Read the model definition and answer for the solid it produces. Units are mm, in the model's axes. A direction names the side the tool comes from. Coordinates: 2 decimals unless noted, no trailing zeros. Order: outer loops, then holes, each group sorted by start corner. A loop starts at its lowest first (then second) coordinate and runs counter-clockwise, first axis right, second up. Notation, with made-up numbers: (-22, 75) - (10, 75) arc R22 cw to (10, 110) - close; hole circle Ø10 at (42.25, -12.5). An arc over 180 degrees is marked (long way). Answer as a JSON object with one key per item and string values. Group by question number.
from build123d import *

# Parameters (mm, degrees)
ESQUISSE1_W        = 95
ESQUISSE1_H        = 75
BOSS_EXTRU_1_DEPTH = 5
BOSS_EXTRU_2_DEPTH = 25
ESQUISSE3_W        = 4.5
ESQUISSE3_H        = 7.5
BOSS_EXTRU_3_DEPTH = 90


with BuildPart() as part:
    # Esquisse1 → Boss.-Extru.1 (new body)
    with BuildSketch(Plane.XY):
        with Locations((47.5, 37.5)):
            Rectangle(ESQUISSE1_W, ESQUISSE1_H)
    extrude(amount=BOSS_EXTRU_1_DEPTH)

    # Esquisse2 → Boss.-Extru.2 (add)
    with BuildSketch(Plane.XY.offset(5)):
        Polygon((0, 70), (0, 75), (95, 75), (95, 0), (0, 0), (0, 5), (90, 5), (90, 70), align=None)
    extrude(amount=BOSS_EXTRU_2_DEPTH)

    # Esquisse3 → Boss.-Extru.3 (add)
    with BuildSketch(Plane.ZY.offset(-90)):
        with Locations((27.75, 66.25)):
            Rectangle(ESQUISSE3_W, ESQUISSE3_H)
        with Locations((27.75, 8.75)):
            Rectangle(ESQUISSE3_W, ESQUISSE3_H)
    extrude(amount=BOSS_EXTRU_3_DEPTH)


solid = part.part
1. For faces 1 (the flat face through (47, 38, 0)), 2 (the flat face through (46, 9, 25.5)), 3 (the flat face through (46, 62.5, 28)), determine the directions among +Z, -Z, +X, -X, +Y, -Y from which every point of the face is accessible in a straight line to the end or side of a thin tool.
2. Straight lines are drawn through the part: L1, parallel to Y at x = 61, z = 17.5; L2, parallel to Z at x = 77, y = 11.5; L3, parallel to X at y = 47.5, z = 13. For each, find the intervals that lie inside material, in ascending order.
3. A cutting plane is placed at C-C on x = 46.5. Write down the section's boundary in (y, z), and give its area (4 significant figures).
4. Given pin 1 (12 mm diameter, centred on x = 18, y = 21.5, fed in from +Z); pin 2 (10 mm diameter, centred on y = 16, z = 20, fed in from -X), each flat-ended and moving along its own axis, determine where each tip first touches the part or whether it passes through.
5. A cutting plane is placed at A-A on y = 8. Write down the section's boundary in (x, z).
6. A cutting plane is placed at B-B on z = 16. Write down the section's boundary in (x, y), and give its area (4 significant figures).
7. For a pull along Y with two mould halves and no side action, classify faces 4 (the flat face through (47, 0, 15)), 5 (the flat face through (46, 12.5, 28)), 6 (the flat face through (0, 38, 4.8)) as pulls with the +Y half, pulls with the -Y half, needs draft (parallel to the pull), parting line crosses it, or undercut.
Derived:
{
 "1": {"face 1": "-Z, +X, -X, +Y, -Y", "face 2": "-X", "face 3": "+Z, -X"},
 "2": {"L1": "y = 0 to 5, 70 to 75", "L2": "z = 0 to 5, 25.5 to 30", "L3": "x = 90 to 95"},
 "3": {"outline": "(0, 0) - (75, 0) - (75, 30) - (62.5, 30) - (62.5, 25.5) - (70, 25.5) - (70, 5) - (5, 5) - (5, 25.5) - (12.5, 25.5) - (12.5, 30) - (0, 30) - close", "area": "692.5 mm2"},
 "4": {"pin 1": "stops at z = 5", "pin 2": "stops at x = 90"},
 "5": {"outline": "(0, 0) - (95, 0) - (95, 30) - (0, 30) - (0, 25.5) - (90, 25.5) - (90, 5) - (0, 5) - close"},
 "6": {"outline": "(0, 0) - (95, 0) - (95, 75) - (0, 75) - (0, 70) - (90, 70) - (90, 5) - (0, 5) - close", "area": "1,275 mm2"},
 "7": {"face 4": "pulls with the -Y half", "face 5": "undercut", "face 6": "needs draft"}
}
